from build123d import *


with BuildPart() as part:
    # Эскиз1 → Повернуть1 (revolve)
    with BuildSketch(Plane.XY, mode=Mode.PRIVATE) as revolve_1_sk:
        Polygon((4.5, 16), (2, 16), (2, 0), (4, 0), (4, 3.5), (4.5, 4), (4.5, 14), (3.5, 14), (3.5, 15), (4.5, 15), align=None)
    revolve_1 = revolve(revolve_1_sk.sketch.rotate(Axis((0, 64.627595022, 0), (0, -1, 0)), 90), axis=Axis((0, 64.627595022, 0), (0, -1, 0)))


with BuildPart() as mirror_1_1:
    # Зеркальное отражение1: Повернуть1 across Top Plane
    add(revolve_1.mirror(Plane(origin=(0, 0, 0), x_dir=(1, 0, 0), z_dir=(0, 1, 0))))


with BuildPart() as part_1:
    add(part.part)

    # Зеркальное отражение1 united with what the copies tou: union Зеркальное отражение1_1
    add(mirror_1_1.part)


solid = part_1.part
Source: CAD feature listing. Evaluate the final solid. Frame: model axes, mm. A direction names the side the tool comes from. Coordinates: 2 decimals unless noted, no trailing zeros. Loops run counter-clockwise (first coordinate to the right, second up) from the corner with the lowest first, then second, coordinate; pieces in that order, holes last. Notation, with made-up numbers: (23, 85) - (57, 85) arc R23 cw to (57, 107) - close; hole circle Ø8 at (47, 71.25). An arc over 180 degrees is marked (long way). One line per item, written item: value. Start each with the question number.
1. Contact query for flat-ended pins moving along their axis: P1, Ø4, axis at y = -1.5, z = 1, coming from the -X side; P2, Ø1, axis at x = 3.5, y = 7, coming from the -Z side; P3, Ø3, axis at x = 0, z = 0, coming from the -Y side. Output: stop coordinate, or through.
2. Mould query, pull axis Y, two halves, no side actions, for faces 3 (the flat face through (2, 16, 1)), 4 (the cylindrical face through (-3.04, -15.51, -3.32)), 5 (the flat face through (4, 14, 0)). Classes: pulls with the +Y half, pulls with the -Y half, needs draft (parallel to the pull), parting line crosses it, or undercut.
3. Set-up query: faces 1 (the cylindrical face through (-3.04, 15.51, -3.32)), 2 (the cylindrical face through (3.905, 0.049, -0.867)). Return all of +Z, -Z, +X, -X, +Y, -Y with unobstructed straight access to the full face (end or side cutting, diameter ignored); none if empty.
4. Section C-C (y = -1). Return the cut outline in (x, z), and give its area (3 significant figures).
5. Section D-D (y = -9). Return the cut outline in (x, z), and give its area (3 significant figures).
6. Ray query, L1, parallel to X at y = 2, z = 0; L2, parallel to X at y = -5, z = 0; L3, parallel to Y at x = -4, z = 0.5. Return the intervals inside material, ascending.
Verdict:
1. P1: stops at x = -4
1. P2: stops at z = -3.35
1. P3: passes through
2. face 3: pulls with the +Y half
2. face 4: needs draft
2. face 5: undercut
3. face 1: +Y, -Y
3. face 2: none
4. outline: circle Ø8 at (0, 0); hole circle Ø4 at (0, 0)
4. area: 37.7 mm2
5. outline: circle Ø9 at (0, 0); hole circle Ø4 at (0, 0)
5. area: 51.1 mm2
6. L1: x = -4 to -2, 2 to 4
6. L2: x = -4.5 to -2, 2 to 4.5
6. L3: y = -16 to -15, -14 to -3.53, 3.53 to 14, 15 to 16
